Geometry: see drawing. Coordinates: mm, zero at the bounding-box minimum. Coordinates: 2 decimals unless noted, no trailing zeros. Loops run counter-clockwise (first coordinate to the right, second up) from the corner with the lowest first, then second, coordinate; pieces in that order, holes last. Notation, with made-up numbers: (13, -14) - (26, -14) arc R18 cw to (26, 8) - close; hole circle Ø4 at (-25.5, 68.5). An arc over 180 degrees is marked (long way). Use a Markdown table: item, result. Add a question column.
1. Section query A-A on y = 11.25. Return the cut outline in (x, z) (1 decimal).
2. Ray query, L1, parallel to Z at x = 571.5, y = 1; L2, parallel to Z at x = 545, y = 4.5; L3, parallel to X at y = 19, z = 101 (1 decimal). Return the intervals inside material, ascending. Write a range as [from, to].
3. Section query B-B on x = 401. Return the cut outline in (y, z) (1 decimal), then the cut area to 3 significant figures.
4. Contact query for flat-ended pins moving along their axis: P1, Ø12, axis at y = 11.5, z = 109, coming from the +X side (1 decimal); P2, Ø1, axis at x = 473, y = 12.5, coming from the -Z side; P3, Ø12, axis at x = 503, y = 15, coming from the -Z side. Output: stop coordinate, or through.
5. Section query C-C on z = 224. Return the cut outline in (x, y).
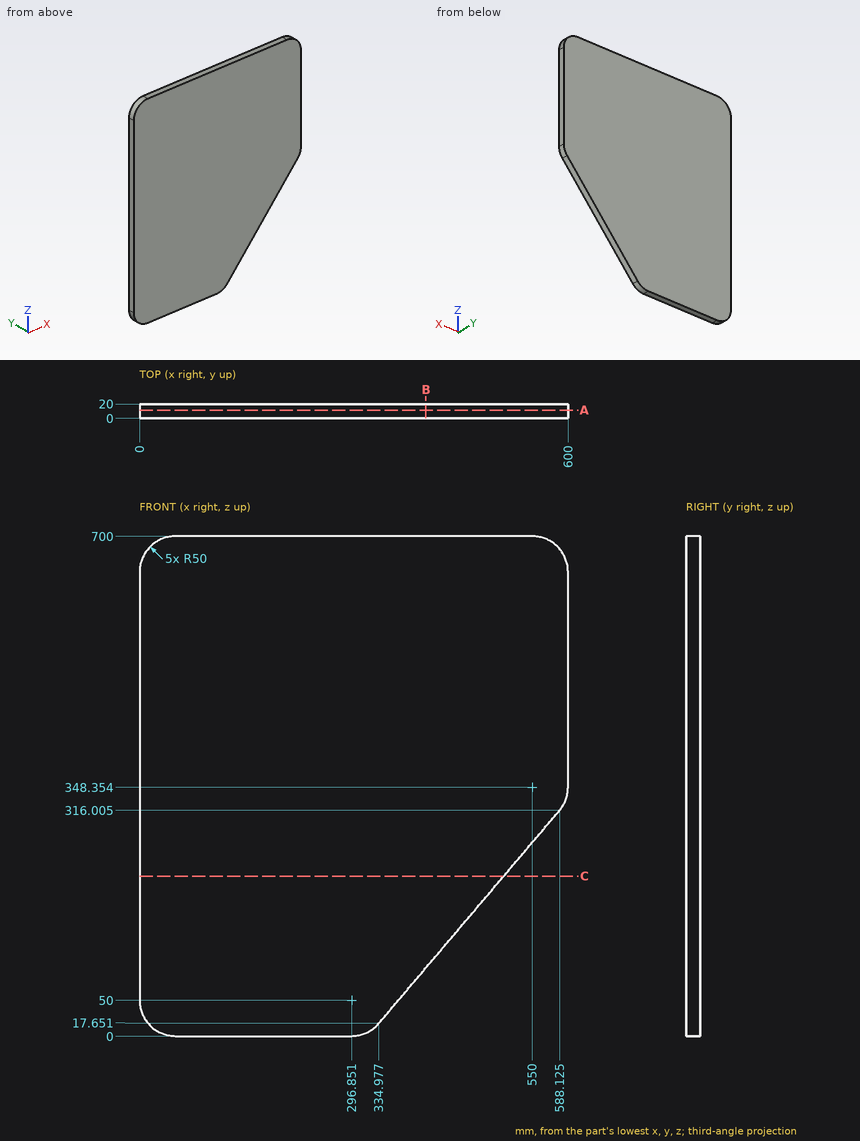
Resolved:
| question | item | result |
|---|---|---|
| 1 | outline | (0, 50) arc R50 ccw to (50, 0) - (296.9, 0) arc R50 ccw to (335, 17.7) - (588.1, 316) arc R50 ccw to (600, 348.4) - (600, 650) arc R50 ccw to (550, 700) - (50, 700) arc R50 ccw to (0, 650) - close |
| 2 | L1 | [296.41, 695.14] |
| 2 | L2 | [265.18, 700] |
| 2 | L3 | [0, 405.7] |
| 3 | outline | (0, 95.5) - (20, 95.5) - (20, 700) - (0, 700) - close |
| 3 | area | 12,100 mm² |
| 4 | P1 | x = 417.6 |
| 4 | P2 | z = 179.73 |
| 4 | P3 | z = 208.61 |
| 5 | outline | (0, 0) - (510.06, 0) - (510.06, 20) - (0, 20) - close |
